Read the model definition and answer for the solid it produces. Units are mm, in the model's axes. Round coordinates to 2 decimals unless told otherwise and drop trailing zeros. Order: outer loops, then holes, each group sorted by start corner. A loop starts at its lowest first (then second) coordinate and runs counter-clockwise, first axis right, second up. Notation, with made-up numbers: (-15.75, 89) -> (11.25, 89) arc R9 cw to (11.25, 93) -> close; hole circle Ø7 at (0, 83.5). An arc over 180 degrees is marked (long way). Use a Markdown table: item, result. Add a question column.
1. Consider L1, parallel to Z at x = -1.05, y = 0; L2, parallel to Z at x = 0.2, y = 0. Determine where each line is inside the solid, lowest interval first. Write a range as [from, to].
2. The mould has two halves that part along Y. Classify faces 1 (the face through (0, 2, 0)), 2 (the face through (2, 2, 1)), 3 (the face through (-1.507, 3.955, -5.158)): +Y half, -Y half, draft (parallel to the pull), parting line (faces both ways), or undercut.
3. Section C-C, the plane x = 1.4 is taken. Give the vertices of the cut face in (y, z), then the cut area to 3 significant figures.
4. Section D-D, the plane x = -0.6 is taken. Give the vertices of the cut face in (y, z), then the cut area to 3 significant figures.
```python
from build123d import *


with BuildPart() as f1:
    # F0 (on Front) → F1 (revolve)
    with BuildSketch(Plane.XZ):
        with BuildLine():
            Line((-2, 2), (0, 2))
            Line((0, 2), (0, 5.5))
            ThreePointArc((0, 5.5), (-0.707107, 5.792893), (-1, 6.5))
            Line((-1, 6.5), (-2, 6.5))
            Line((-2, 6.5), (-2, 4.5))
            Line((-2, 4.5), (-1.85, 4.5))
            ThreePointArc((-1.85, 4.5), (-2, 3.75), (-1.85, 3))
            Line((-1.85, 3), (-2, 3))
            Line((-2, 3), (-2, 2))
        make_face()
    revolve(axis=Axis((-0.379604, 0, 0), (1, 0, 0)))

    # F2: F1 across face


with BuildPart() as f1_1:
    add(f1.part)
    add(f1.part.mirror(Plane.YZ))


solid = f1_1.part
```
Verdict:
| question | item | result |
|---|---|---|
| 1 | L1 | z = [-6.5, -2], [2, 6.5] |
| 1 | L2 | z = [-5.52, -2], [2, 5.52] |
| 2 | face 1 | undercut |
| 2 | face 2 | draft |
| 2 | face 3 | parting line |
| 3 | outline | circle Ø13 at (0, 0); hole circle Ø4 at (0, 0) |
| 3 | area | 120 mm2 |
| 4 | outline | circle Ø11.4 at (0, 0); hole circle Ø4 at (0, 0) |
| 4 | area | 89.5 mm2 |
